Here's how the part is built. I have some questions about the finished solid (model axes, mm). A direction names the side the tool comes from. Coordinates: 2 decimals unless noted, no trailing zeros. Write each loop counter-clockwise with the first axis right and the second up, starting at its lowest first coordinate (ties: lowest second). Pieces come first, ordered by that corner, then holes.
Item 1: If we section it at C-C (x = -7): Please give me the cut outline in (y, z), then the cut area to 3 significant figures.
Item 2: If we section it at B-B (y = 0.4): Please give me the cut outline in (x, z).
Item 3: I'm going to push flat-ended pins straight in: pin 1 Ø5 at (x, z) = (7, 5) entering from -Y; pin 2 Ø0.6 at (x, y) = (-0.5, 1.5) entering from +Z; pin 3 Ø1 at (x, y) = (0, 1.5) entering from -Z. Where does each tip first touch, or does it pass through?
Item 4: If we section it at D-D (z = 5): Please give me the cut outline in (x, y).
Item 5: We'd pull the mould along X, two halves only. Please class faces 1 (the face through (-11, 1, 0)), 2 (the face through (-6, 1, 10)), 3 (the face through (0, 1, 7.5)): +X half, -X half, draft (parallel to the pull), parting line (faces both ways), or undercut.
Item 6: For faces 4 (the face through (-3, 2, 0)), 5 (the face through (1, 1, -9)), 6 (the face through (-1, 1, 9)), 7 (the face through (0, 1, 2.5)), 8 (the face through (11, 1, 0)), which set-ups out of +Z, -Z, +X, -X, +Y, -Y let a thin tool reach every point of the face, with its end or its side?
Item 7: If I drill on line 1 (X direction, y = 0.9, z = 5); line 2 (X direction, y = 0.35, z = -5.75); line 3 (X direction, y = 0.65, z = 1.25), over which ranges is the centre line in solid material (lowest first)?
Item 8: If we section it at A-A (z = -1.75): Please give me the cut outline in (x, y).
from build123d import *

# Parameters (mm, degrees)
SKETCH1_W           = 22
SKETCH1_H           = 20
BOSS_EXTRUDE1_DEPTH = 2
SKETCH2_R           = 1.5
SKETCH2_W           = 2
SKETCH2_H           = 2.5
SKETCH2_H_2         = 5
CUT_EXTRUDE1_DEPTH  = 2


with BuildPart() as part:
    # Sketch1 → Boss-Extrude1 (new body)
    with BuildSketch(Plane(origin=(0, 0, 0), x_dir=(1, 0, 0), z_dir=(0, 1, 0))):
        Rectangle(SKETCH1_W, SKETCH1_H)
    extrude(amount=BOSS_EXTRUDE1_DEPTH)

    # Sketch2 → Cut-Extrude1 (cut)
    with BuildSketch(Plane(origin=(0, 2, 0), x_dir=(1, 0, 0), z_dir=(0, 1, 0))):
        with Locations(Location((-7, 5, 0), (0, 0, 270))):
            Circle(SKETCH2_R)
        with Locations(Location((-7, -5, 0), (0, 0, 270))):
            Circle(SKETCH2_R)
        with Locations(Location((7, 5, 0), (0, 0, 270))):
            Circle(SKETCH2_R)
        with Locations(Location((7, -5, 0), (0, 0, 270))):
            Circle(SKETCH2_R)
        with Locations((0, 8.75)):
            Rectangle(SKETCH2_W, SKETCH2_H)
        Rectangle(SKETCH2_W, SKETCH2_H_2)
        with Locations((0, -8.75)):
            Rectangle(SKETCH2_W, SKETCH2_H)
    extrude(amount=-CUT_EXTRUDE1_DEPTH, mode=Mode.SUBTRACT)


solid = part.part
Answer list:
1. outline: (0, -10) - (2, -10) - (2, -6.5) - (0, -6.5) - close; (0, -3.5) - (2, -3.5) - (2, 3.5) - (0, 3.5) - close; (0, 6.5) - (2, 6.5) - (2, 10) - (0, 10) - close
1. area: 28.0 mm2
2. outline: (-11, -10) - (-1, -10) - (-1, -7.5) - (1, -7.5) - (1, -10) - (11, -10) - (11, 10) - (1, 10) - (1, 7.5) - (-1, 7.5) - (-1, 10) - (-11, 10) - close; hole circle Ø3 at (-7, -5); hole circle Ø3 at (-7, 5); hole (-1, -2.5) - (1, -2.5) - (1, 2.5) - (-1, 2.5) - close; hole circle Ø3 at (7, -5); hole circle Ø3 at (7, 5)
3. pin 1: stops at y = 0
3. pin 2: stops at z = 7.5
3. pin 3: stops at z = -7.5
4. outline: (-11, 0) - (-8.5, 0) - (-8.5, 2) - (-11, 2) - close; (-5.5, 0) - (5.5, 0) - (5.5, 2) - (-5.5, 2) - close; (8.5, 0) - (11, 0) - (11, 2) - (8.5, 2) - close
5. face 1: -X half
5. face 2: draft
5. face 3: undercut
6. face 4: +Z, -Z, +X, -X, +Y
6. face 5: -Z, +Y, -Y
6. face 6: +Z, +Y, -Y
6. face 7: +Y, -Y
6. face 8: +Z, -Z, +X, +Y, -Y
7. line 1: x = -11 to -8.5, -5.5 to 5.5, 8.5 to 11
7. line 2: x = -11 to -8.3, -5.7 to 5.7, 8.3 to 11
7. line 3: x = -11 to -1, 1 to 11
8. outline: (-11, 0) - (-1, 0) - (-1, 2) - (-11, 2) - close; (1, 0) - (11, 0) - (11, 2) - (1, 2) - close
